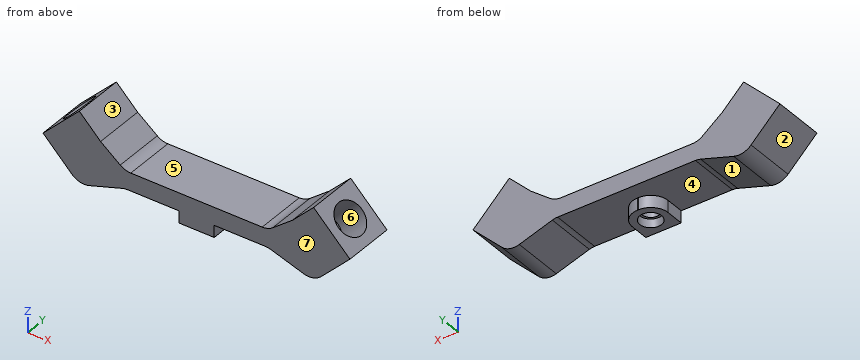
from build123d import *

# Parameters (mm, degrees)
BOSS_EXTRUDE1_DEPTH = 38.1
SKETCH2_R           = 12.065
CUT_EXTRUDE1_DEPTH  = 25.4
SKETCH7_R           = 12.065
CUT_EXTRUDE2_DEPTH  = 25.4
SKETCH9_W           = 26.289
SKETCH9_H           = 26.289
BOSS_EXTRUDE3_DEPTH = 8.89
SKETCH10_R          = 8.0645
CUT_EXTRUDE3_DEPTH  = 6.35
SKETCH12_R          = 6.35
CUT_EXTRUDE5_DEPTH  = 5.08
FILLET1_R           = 12.7


with BuildPart() as part:
    # Sketch1 → Boss-Extrude1 (new body)
    with BuildSketch(Plane(origin=(0, 0, 0), x_dir=(1, 0, 0), z_dir=(0, 1, 0))):
        with BuildLine():
            Line((-8.394951703, 35.720764917), (16.107614613, 27.828435078))
            ThreePointArc((16.107614613, 27.828435078), (18.03059142, 27.370657964), (20.001310729, 27.216823331))
            Line((20.001310729, 27.216823331), (122.238689271, 27.216823331))
            ThreePointArc((122.238689271, 27.216823331), (124.20940858, 27.370657964), (126.132385387, 27.828435078))
            Line((126.132385387, 27.828435078), (150.634951703, 35.720764917))
            ThreePointArc((150.634951703, 35.720764917), (157.509150211, 35.977683688), (163.508903941, 32.612632786))
            Line((163.508903941, 32.612632786), (184.96230509, 11.159231637))
            Line((184.96230509, 11.159231637), (158.021536726, -15.781536726))
            Line((158.021536726, -15.781536726), (142.24, 0))
            Line((142.24, 0), (127.676821583, 11.356327171))
            ThreePointArc((127.676821583, 11.356327171), (123.996342172, 13.351360126), (119.867179962, 14.041363479))
            Line((119.867179962, 14.041363479), (22.372820038, 14.041363479))
            ThreePointArc((22.372820038, 14.041363479), (18.243657828, 13.351360126), (14.563178417, 11.356327171))
            Line((14.563178417, 11.356327171), (0, 0))
            Line((0, 0), (-15.781536726, -15.781536726))
            Line((-15.781536726, -15.781536726), (-42.72230509, 11.159231637))
            Line((-42.72230509, 11.159231637), (-21.268903941, 32.612632786))
            ThreePointArc((-21.268903941, 32.612632786), (-15.269150211, 35.977683688), (-8.394951703, 35.720764917))
        make_face()
    extrude(amount=BOSS_EXTRUDE1_DEPTH)

    # Sketch2 → Cut-Extrude1 (cut)
    with BuildSketch(Plane(origin=(-15.781536726, 0, 15.781536726), x_dir=(0.7071067811865477, 0, 0.7071067811865475), z_dir=(-0.7071067811865475, 0, 0.7071067811865477))):
        with Locations((-19.05, 19.05)):
            Circle(SKETCH2_R)
    extrude(amount=-CUT_EXTRUDE1_DEPTH, mode=Mode.SUBTRACT)

    # Sketch7 → Cut-Extrude2 (cut)
    with BuildSketch(Plane(origin=(86.901536726, 0, 86.901536726), x_dir=(0.7071067811865472, 0, -0.7071067811865478), z_dir=(0.7071067811865478, 0, 0.7071067811865472))):
        with Locations((119.628868556, 19.05)):
            Circle(SKETCH7_R)
    extrude(amount=-CUT_EXTRUDE2_DEPTH, mode=Mode.SUBTRACT)

    # Sketch9 → Boss-Extrude3 (add)
    with BuildSketch(Plane(origin=(0, 0, -27.216823331), x_dir=(-1, 0, 0), z_dir=(0, 0, -1))):
        with Locations((-71.12, 13.1445)):
            Rectangle(SKETCH9_W, SKETCH9_H)
    extrude(amount=BOSS_EXTRUDE3_DEPTH)

    # Sketch10 → Cut-Extrude3 (cut)
    with BuildSketch(Plane(origin=(0, 0, -36.106823331), x_dir=(-1, 0, 0), z_dir=(0, 0, -1))):
        with Locations((-71.12, 13.1445)):
            Circle(SKETCH10_R)
    extrude(amount=-CUT_EXTRUDE3_DEPTH, mode=Mode.SUBTRACT)

    # Sketch12 → Cut-Extrude5 (cut)
    with BuildSketch(Plane(origin=(0, 0, -29.756823331), x_dir=(-1, 0, 0), z_dir=(0, 0, -1))):
        with Locations((-71.12, 13.1445)):
            Circle(SKETCH12_R)
    extrude(amount=-CUT_EXTRUDE5_DEPTH, mode=Mode.SUBTRACT)

    # Fillet1
    fillet1_edges = [part.edges().sort_by_distance(p)[0] for p in [
        (57.9755, 26.289, -31.661823331),
        (84.2645, 26.289, -31.661823331),
    ]]
    fillet(fillet1_edges, radius=FILLET1_R)


solid = part.part
Work out the finished part from the listing and answer in its coordinate system (mm). Face numbers are marked on the shaded views. A direction names the side the tool comes from. Round coordinates to 2 decimals unless told otherwise and drop trailing zeros. Write each loop counter-clockwise with the first axis right and the second up, starting at its lowest first coordinate (ties: lowest second). Pieces come first, ordered by that corner, then holes.
1) The mould has two halves that part along Y. Classify the marked faces 5, 6 and 7: pulls with the +Y half, pulls with the -Y half, needs draft (parallel to the pull), parting line crosses it, or undercut.
2) Straight lines are drawn through the part: line 1 (X direction, y = 25.5, z = -22.5); line 2 (Y direction, x = 71.12, z = -28.2); line 3 (Z direction, x = 120, y = 32). For each, find the intervals that lie inside material, in ascending order.
3) A cutting plane is placed at B-B (x = 7). Give the vertices of the cut face in (y, z).
4) A cutting plane is placed at A-A (x = 114). Give the vertices of the cut face in (y, z), plus the area to 3 significant figures.
5) A tool of negligible diameter and unlimited length cuts with its end or side. For the marked faces 1, 2, 3 and 4, from which of +Z, -Z, +X, -X, +Y, -Y can it reach the whole face along a straight path? Write none if from no direction.
6) Given pin 1 Ø10 at (y, z) = (7, 5.5) entering from +X; pin 2 Ø4 at (x, y) = (146, 26) entering from -Z; pin 3 Ø1 at (y, z) = (15, -23.5) entering from -X; pin 4 Ø3 at (x, z) = (95.5, -11) entering from +Y, each flat-ended and moving along its own axis, determine where each tip first touches the part or whether it passes through.
Completed:
1. face 5: needs draft
1. face 6: undercut
1. face 7: pulls with the -Y half
2. line 1: x = -31.38 to -18.86, -18.14 to 160.38, 161.1 to 173.62
2. line 2: y = 0 to 6.79, 19.49 to 26.29
2. line 3: z = -27.22 to -14.04
3. outline: (0, -30.76) - (38.1, -30.76) - (38.1, -5.46) - (0, -5.46) - close
4. outline: (0, -27.22) - (38.1, -27.22) - (38.1, -14.04) - (0, -14.04) - close
4. area: 502 mm2
5. face 1: -Z, +Y, -Y
5. face 2: -Z, -X, +Y, -Y
5. face 3: +Z, +Y, -Y
5. face 4: -Z, +Y
6. pin 1: stops at x = 173.3
6. pin 2: stops at z = -34.87
6. pin 3: stops at x = -30.88
6. pin 4: passes through
